The model under review builds one solid part; all positions refer to its coordinate system, in mm. A direction names the side the tool comes from. Coordinates: 2 decimals unless noted, no trailing zeros. Write each loop counter-clockwise with the first axis right and the second up, starting at its lowest first coordinate (ties: lowest second). Pieces come first, ordered by that corner, then holes. Notation, with made-up numbers: (67.5, 2.5) - (71.5, 2.5) arc R26 cw to (71.5, 33.5) - close; hole circle Ø3 at (-15, 35.25). An arc over 180 degrees is marked (long way). Put each result on its own line as item: value.
from build123d import *

# Parameters (mm, degrees)
F0_W      = 108
F0_H      = 130
F1_DEPTH  = 90
F2_R      = 6.5
F3_DEPTH  = 90.001
F4_W      = 108
F4_H      = 80
F5_DEPTH  = 25
F6_W      = 90
F6_H      = 50
F7_DEPTH  = 25
F8_R      = 10
F9_DEPTH  = 20
F10_R     = 10
F11_DEPTH = 20
F12_W     = 20
F12_H     = 55
F12_W_2   = 44
F12_H_2   = 20
F13_DEPTH = 5
F15_ANGLE = 180


with BuildPart() as f1:
    # F0 (on Right) → F1 (new body)
    with BuildSketch(Plane.YZ):
        Rectangle(F0_W, F0_H)
    extrude(amount=-F1_DEPTH)

    # F2 (on face) → F3 (cut, through all)
    with BuildSketch(Plane(origin=(-90, 0, 0), x_dir=(0, -1, 0), z_dir=(-1, 0, 0))):
        with Locations((-42, 47)):
            Circle(F2_R)
        with Locations((42, 47)):
            Circle(F2_R)
        with Locations((-42, -47)):
            Circle(F2_R)
        with Locations((42, -47)):
            Circle(F2_R)
    extrude(amount=-F3_DEPTH, mode=Mode.SUBTRACT)

    # F4 (on face) → F5 (cut)
    with BuildSketch(Plane(origin=(-90, 0, 0), x_dir=(0, -1, 0), z_dir=(-1, 0, 0))):
        with Locations((0, -25)):
            Rectangle(F4_W, F4_H)
    extrude(amount=-F5_DEPTH, mode=Mode.SUBTRACT)

    # F6 (on face) → F7 (cut)
    with BuildSketch(Plane.XY.offset(65)):
        with Locations((-45, 0)):
            Rectangle(F6_W, F6_H)
    extrude(amount=-F7_DEPTH, mode=Mode.SUBTRACT)

    # F8 (on face) → F9 (cut)
    with BuildSketch(Plane(origin=(-65, 0, 0), x_dir=(0, -1, 0), z_dir=(-1, 0, 0))):
        with Locations((42, -47)):
            Circle(F8_R)
        with Locations((-42, -47)):
            Circle(F8_R)
    extrude(amount=-F9_DEPTH, mode=Mode.SUBTRACT)

    # F10 (on face) → F11 (cut)
    with BuildSketch(Plane(origin=(-90, 0, 0), x_dir=(0, -1, 0), z_dir=(-1, 0, 0))):
        with Locations((42, 47)):
            Circle(F10_R)
        with Locations((-42, 47)):
            Circle(F10_R)
    extrude(amount=-F11_DEPTH, mode=Mode.SUBTRACT)

    # F12 (on face) → F13 (cut)
    with BuildSketch(Plane.YZ):
        with Locations((0, -37.5)):
            Rectangle(F12_W, F12_H)
        with Locations((-32, 0)):
            Rectangle(F12_W_2, F12_H_2)
        Rectangle(F12_W, F12_H_2)
        with Locations((32, 0)):
            Rectangle(F12_W_2, F12_H_2)
        with Locations((0, 37.5)):
            Rectangle(F12_W, F12_H)
    extrude(amount=-F13_DEPTH, mode=Mode.SUBTRACT)


with BuildPart() as f1_1:
    # F15: moved
    add(f1.part.rotate(Axis((42.7994653583, 0, 0), (1, 0, 0)), F15_ANGLE))


solid = f1_1.part
1. Consider section C-C on z = -47. State the section outline as (x, y) points.
Determined:
outline: (-90, -54) - (0, -54) - (0, -48.5) - (-70, -48.5) - (-70, -52) - (-90, -52) - close; (-90, -32) - (-70, -32) - (-70, -35.5) - (0, -35.5) - (0, -25) - (-90, -25) - close; (-90, 25) - (0, 25) - (0, 35.5) - (-70, 35.5) - (-70, 32) - (-90, 32) - close; (-90, 52) - (-70, 52) - (-70, 48.5) - (0, 48.5) - (0, 54) - (-90, 54) - close
2. To check wall thickness, follow probe 1 along Z at (x, y) = (-29.5, -42); probe 2 along Z at (x, y) = (-59, 42); probe 3 along Y at (x, z) = (-86, -49). State the ranges of each line that lie inside material, in increasing order.
Determined:
probe 1: z = -65 to -53.5, -40.5 to 40.5, 53.5 to 65
probe 2: z = -65 to -53.5, -40.5 to 37, 57 to 65
probe 3: y = -54 to -51.8, -32.2 to -25, 25 to 32.2, 51.8 to 54
3. Consider section D-D on y = 42. State the section outline as (x, z) points, plus the area to 4 significant figures.
Determined:
outline: (-90, -65) - (0, -65) - (0, -53.5) - (-70, -53.5) - (-70, -57) - (-90, -57) - close; (-90, -37) - (-70, -37) - (-70, -40.5) - (0, -40.5) - (0, -10) - (-5, -10) - (-5, 10) - (0, 10) - (0, 40.5) - (-45, 40.5) - (-45, 37) - (-65, 37) - (-65, -15) - (-90, -15) - close; (-65, 57) - (-45, 57) - (-45, 53.5) - (0, 53.5) - (0, 65) - (-65, 65) - close
area: 7,305 mm^2
4. Machinability: for faces 5 (the flat face through (-2, -10, 38)), 6 (the flat face through (-45, 42, 54)), 7 (the flat face through (-46, -25, -53)), 8 (the flat face through (-78, -1, -15)), which of the approach directions +Z, -Z, +X, -X, +Y, -Y give a long, thin tool a straight path to every point of the face, cutting with its end or side? Answer none if there is none.
Determined:
face 5: +Z, -Z, +X
face 6: -X
face 7: -Z, +X, -X
face 8: +Z, -X, +Y, -Y
5. For pin 1 Ø6 at (y, z) = (-38.5, -47.5) entering from -X; pin 2 Ø10 at (y, z) = (-31.5, -11.5) entering from +X; pin 3 Ø1 at (x, y) = (-79.5, 14.5) entering from +Z; pin 4 Ø17 at (y, z) = (-42, 47) entering from -X, all flat-tipped, find the tip position at first contact; note any pin that passes through.
Determined:
pin 1: stops at x = -70
pin 2: stops at x = 0
pin 3: stops at z = -15
pin 4: stops at x = -45
6. The part is to be moulded in two halves that separate along Z. For faces 1 (the flat face through (-46, 0, -40)), 2 (the flat face through (-2, 32, -10)), 3 (the flat face through (-45, -42, 54)), 4 (the flat face through (-34, 54, 1)), say which applies: +Z half, -Z half, draft (parallel to the pull), parting line (faces both ways), or undercut.
Determined:
face 1: -Z half
face 2: undercut
face 3: undercut
face 4: draft
7. Consider section B-B on x = -19. State the section outline as (y, z) points.
Determined:
outline: (-54, -65) - (-25, -65) - (-25, -40) - (25, -40) - (25, -65) - (54, -65) - (54, 65) - (-54, 65) - close; hole circle Ø13 at (-42, -47); hole circle Ø13 at (-42, 47); hole circle Ø13 at (42, -47); hole circle Ø13 at (42, 47)
8. Consider section A-A on z = 47. State the section outline as (x, y) points, plus the area to 3 significant figures.
Determined:
outline: (-65, -54) - (0, -54) - (0, -48.5) - (-45, -48.5) - (-45, -52) - (-65, -52) - close; (-65, -32) - (-45, -32) - (-45, -35.5) - (0, -35.5) - (0, -10) - (-5, -10) - (-5, 10) - (0, 10) - (0, 35.5) - (-45, 35.5) - (-45, 32) - (-65, 32) - close; (-65, 52) - (-45, 52) - (-45, 48.5) - (0, 48.5) - (0, 54) - (-65, 54) - close
area: 4,950 mm^2
